```python
from build123d import *

# Parameters (mm, degrees)
MODEL_W                 = 3
MODEL_H                 = 3
SALIENTE_EXTRUIR1_DEPTH = 3


with BuildPart() as part:
    # Model → Saliente-Extruir1 (new body)
    with BuildSketch(Plane.XY):
        with BuildLine():
            Line((9.904781567, 296.774995526), (126.904781567, 296.774995526))
            ThreePointArc((126.904781567, 296.774995526), (131.404781567, 292.274995526), (126.904781567, 287.774995526))
            Line((126.904781567, 287.774995526), (9.904781567, 287.774995526))
            ThreePointArc((9.904781567, 287.774995526), (5.404781567, 292.274995526), (9.904781567, 296.774995526))
        make_face()
        with Locations((9.904781567, 292.274995526)):
            Rectangle(MODEL_W, MODEL_H, mode=Mode.SUBTRACT)
        with Locations((18.904781567, 292.274995526)):
            Rectangle(MODEL_W, MODEL_H, mode=Mode.SUBTRACT)
        with Locations((27.904781567, 292.274995526)):
            Rectangle(MODEL_W, MODEL_H, mode=Mode.SUBTRACT)
        with Locations((36.904781567, 292.274995526)):
            Rectangle(MODEL_W, MODEL_H, mode=Mode.SUBTRACT)
        with Locations((45.904781567, 292.274995526)):
            Rectangle(MODEL_W, MODEL_H, mode=Mode.SUBTRACT)
        with Locations((54.904781567, 292.274995526)):
            Rectangle(MODEL_W, MODEL_H, mode=Mode.SUBTRACT)
        with Locations((63.904781567, 292.274995526)):
            Rectangle(MODEL_W, MODEL_H, mode=Mode.SUBTRACT)
        with Locations((72.904781567, 292.274995526)):
            Rectangle(MODEL_W, MODEL_H, mode=Mode.SUBTRACT)
        with Locations((81.904781567, 292.274995526)):
            Rectangle(MODEL_W, MODEL_H, mode=Mode.SUBTRACT)
        with Locations((90.904781567, 292.274995526)):
            Rectangle(MODEL_W, MODEL_H, mode=Mode.SUBTRACT)
        with Locations((126.904781567, 292.274995526)):
            Rectangle(MODEL_W, MODEL_H, mode=Mode.SUBTRACT)
        with Locations((99.904781567, 292.274995526)):
            Rectangle(MODEL_W, MODEL_H, mode=Mode.SUBTRACT)
        with Locations((108.904781567, 292.274995526)):
            Rectangle(MODEL_W, MODEL_H, mode=Mode.SUBTRACT)
        with Locations((117.904781567, 292.274995526)):
            Rectangle(MODEL_W, MODEL_H, mode=Mode.SUBTRACT)
    extrude(amount=SALIENTE_EXTRUIR1_DEPTH)


solid = part.part
```
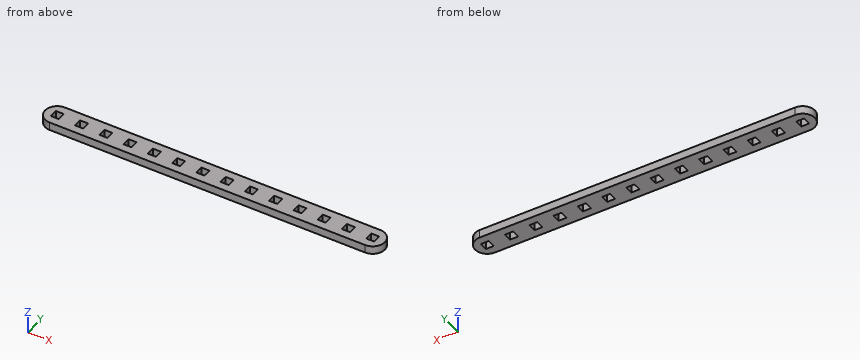
Geometry: final body of the model. Coordinates: model frame, mm. Round coordinates to 2 decimals unless told otherwise and drop trailing zeros.
Item 1: Pin query (flat end, axial travel): P1, Ø0.9, axis at y = 291.5, z = 1.5, coming from the -X side; P2, Ø1.5, axis at y = 290, z = 0.5, coming from the +X side. Return the tip coordinate at first contact, or that it passes through.
Item 2: Material intervals for L1, parallel to Y at x = 100.5, z = 0.75 (3 decimals); L2, parallel to X at y = 288.75, z = 0.5; L3, parallel to X at y = 295, z = 2.5, sorted ascending.
Item 3: Section query A-A (z = 0.8). Give the number of separate pieces and of enclosed holes in the cut face, plus the area to 3 significant figures.
Completed:
1. P1: stops at x = 5.42
1. P2: stops at x = 131.14
2. L1: y = 287.775 to 290.775, 293.775 to 296.775
2. L2: x = 7.11 to 129.7
2. L3: x = 6.32 to 130.49
3. separate pieces: 1
3. enclosed holes: 14
3. area: 991 mm2
